from build123d import *

# Parameters (mm, degrees)
SKETCH1_R           = 1.650000007
BOSS_EXTRUDE1_DEPTH = 1
SKETCH7_R           = 1.6
CUT_EXTRUDE2_DEPTH  = 2


with BuildPart() as part:
    # Sketch1 → Boss-Extrude1 (new, symmetric)
    with BuildSketch(Plane(origin=(0, 0, 0), x_dir=(1, 0, 0), z_dir=(0, 1, 0))):
        with BuildLine():
            Line((-56.656859897, 90.483506167), (-36.993673105, 86.828497938))
            ThreePointArc((-36.993673105, 86.828497938), (-33.173282872, 84.013663947), (-34.729774781, 79.530807173))
            Line((-34.729774781, 79.530807173), (-58.047969803, 63.522628609))
            ThreePointArc((-58.047969803, 63.522628609), (-61.213536363, 62.923269927), (-63.79414326, 64.852132418))
            ThreePointArc((-63.79414326, 64.852132418), (-64.662572796, 65.817505246), (-65.857598376, 66.32547022))
            Line((-65.857598376, 66.32547022), (-94.996570641, 71.741844715))
            ThreePointArc((-94.996570641, 71.741844715), (-96.92158748, 72.993398991), (-97.397797425, 75.239573968))
            Line((-97.397797425, 75.239573968), (-94.29104043, 91.953282742))
            ThreePointArc((-94.29104043, 91.953282742), (-93.039486154, 93.878299581), (-90.793311177, 94.354509526))
            Line((-90.793311177, 94.354509526), (-61.654338999, 88.938135048))
            ThreePointArc((-61.654338999, 88.938135048), (-60.356600681, 88.982743171), (-59.199275822, 89.571567253))
            ThreePointArc((-59.199275822, 89.571567253), (-58.007370108, 90.248625312), (-56.656859897, 90.483506167))
        make_face()
        with Locations(Location((-56.656859897, 86.483506167, 0), (0, 0, 270))):
            Circle(SKETCH1_R, mode=Mode.SUBTRACT)
        with Locations(Location((-36.993673105, 82.828497938, 0), (0, 0, 270))):
            Circle(SKETCH1_R, mode=Mode.SUBTRACT)
        with Locations(Location((-60.311868127, 66.820319374, 0), (0, 0, 270))):
            Circle(SKETCH1_R, mode=Mode.SUBTRACT)
    extrude(amount=BOSS_EXTRUDE1_DEPTH, both=True)

    # Sketch7 → Cut-Extrude2 (cut)
    with BuildSketch(Plane(origin=(0, 1, 0), x_dir=(1, 0, 0), z_dir=(0, 1, 0))):
        with Locations(Location((-88.848960421, 88.398881924, 0), (0, 0, 270))):
            Circle(SKETCH7_R)
        with Locations(Location((-91.041965359, 76.600969848, 0), (0, 0, 270))):
            Circle(SKETCH7_R)
        with Locations(Location((-75.084729666, 85.840376163, 0), (0, 0, 270))):
            Circle(SKETCH7_R)
        with Locations(Location((-77.277734604, 74.042464088, 0), (0, 0, 270))):
            Circle(SKETCH7_R)
    extrude(amount=-CUT_EXTRUDE2_DEPTH, mode=Mode.SUBTRACT)


solid = part.part
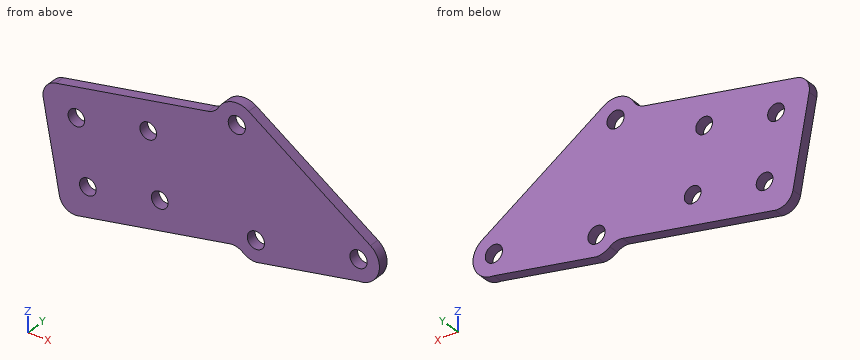
Build history of the part. All positions in model axes, mm. Coordinates: 2 decimals unless noted, no trailing zeros. Order: outer loops, then holes, each group sorted by start corner. A loop starts at its lowest first (then second) coordinate and runs counter-clockwise, first axis right, second up. Notation, with made-up numbers: (47, 85) - (67, 85) arc R23 cw to (67, 124) - close; hole circle Ø5 at (59.5, 32.5). An arc over 180 degrees is marked (long way). Write item = value, one per line. Start each with the question number.
1) Saw through at B-B on y = -0.7. Write the cut outline in (x, z).
2) Saw through at A-A on z = -77. Write the cut outline in (x, y).
3) Wall check: line 1 along X through (y, z) = (0.6, -86); line 2 along Z through (x, y) = (-56.5, -0.1); line 3 along Z through (x, y) = (-38.5, 0.9). Give the ranges that are in metal, low to high. Write a range as from..to.
4) Saw through at D-D on x = -44. Write the cut outline in (y, z).
5) Saw through at C-C on x = -65. Write the cut outline in (y, z).
6) Flat gauge pins, fed straight in: pin 1 Ø2.5 at (x, z) = (-60.31, -66.82) entering from -Y; pin 2 Ø3.5 at (x, z) = (-77.28, -74.04) entering from +Y. Where does each tip first touch, or does it go through?
From the geometry:
q1.outline = (-97.4, -75.24) - (-94.29, -91.95) arc R3 ccw to (-90.79, -94.35) - (-61.65, -88.94) arc R3 cw to (-59.2, -89.57) arc R4 ccw to (-56.66, -90.48) - (-36.99, -86.83) arc R4 ccw to (-34.73, -79.53) - (-58.05, -63.52) arc R4 ccw to (-63.79, -64.85) arc R3 cw to (-65.86, -66.33) - (-95, -71.74) arc R3 ccw to start; hole circle Ø3.2 at (-91.04, -76.6); hole circle Ø3.2 at (-88.85, -88.4); hole circle Ø3.2 at (-77.28, -74.04); hole circle Ø3.2 at (-75.08, -85.84); hole circle Ø3.3 at (-60.31, -66.82); hole circle Ø3.3 at (-56.66, -86.48); hole circle Ø3.3 at (-36.99, -82.83)
q2.outline = (-97.07, -1) - (-92.59, -1) - (-92.59, 1) - (-97.07, 1) - close; (-89.49, -1) - (-38.42, -1) - (-38.42, 1) - (-89.49, 1) - close
q3.line_1 = -95.4..-76.68, -73.49..-58.23, -55.08..-34.56
q3.line_2 = -90.45..-88.13, -84.84..-64.59
q3.line_3 = -87.11..-83.5, -82.16..-76.94
q4.outline = (-1, -88.13) - (1, -88.13) - (1, -73.17) - (-1, -73.17) - close
q5.outline = (-1, -89.56) - (1, -89.56) - (1, -66.03) - (-1, -66.03) - close
q6.pin_1 = through
q6.pin_2 = 1
